from build123d import *

# Parameters (mm, degrees)
F0_W     = 140
F0_H     = 60
F1_DEPTH = 60
F2_R     = 10
F3_DEPTH = 20
F4_R     = 10
F5_DEPTH = 65
F6_R     = 10
F7_DEPTH = 20


with BuildPart() as f1:
    # F0 (on Front) → F1 (new body)
    with BuildSketch(Plane.XZ):
        Rectangle(F0_W, F0_H)
    extrude(amount=F1_DEPTH)

    # F2 (on face) → F3 (join)
    with BuildSketch(Plane.XY.offset(30)):
        with Locations((-40, -30)):
            Circle(F2_R)
    extrude(amount=F3_DEPTH)

    # F4 (on face) → F5 (cut)
    with BuildSketch(Plane.XY.offset(30)):
        with Locations((0, -30)):
            Circle(F4_R)
    extrude(amount=-F5_DEPTH, mode=Mode.SUBTRACT)

    # F6 (on face) → F7 (cut)
    with BuildSketch(Plane.XY.offset(30)):
        with Locations((40, -30)):
            Circle(F6_R)
    extrude(amount=-F7_DEPTH, mode=Mode.SUBTRACT)


solid = f1.part
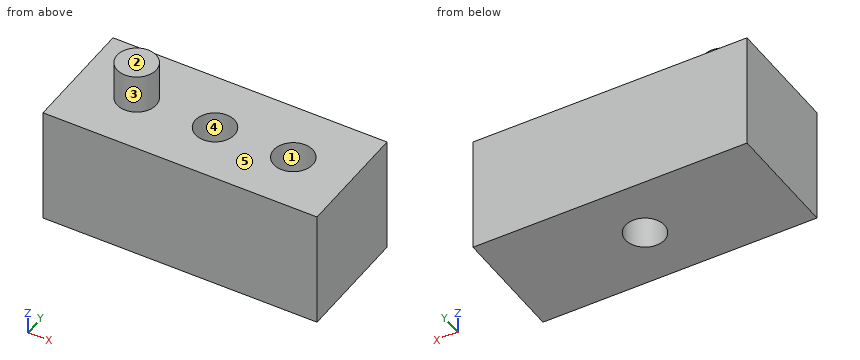
Model file for the job. Use its own axes, mm. Face numbers are marked on the shaded views. A direction names the side the tool comes from. Coordinates: 2 decimals unless noted, no trailing zeros. Write each loop counter-clockwise with the first axis right and the second up, starting at its lowest first coordinate (ties: lowest second). Pieces come first, ordered by that corner, then holes. Notation, with made-up numbers: (19, 79.5) -> (42, 79.5) arc R26 ccw to (42, 102.5) -> close; hole circle Ø10 at (-12, 41.5). An arc over 180 degrees is marked (long way). One line per item, written item: value. Start each with the question number.
1) Probe probe 1 along Y at (x, z) = (40, 19.75); probe 2 along Z at (x, y) = (-47.5, -3); probe 3 along X at (y, z) = (-26, 34). List the from-to ranges inside material, lowest first.
2) Pull direction X, two halves, no side cores. Call the marked faces 3, 4 and 5: +X half, -X half, draft (parallel to the pull), parting line (faces both ways), or undercut.
3) Slice it at B-B on y = -30. Write the cut outline in (x, z), then the cut area to 3 significant figures.
4) Flat gauge pins, fed straight in: pin 1 Ø6 at (x, z) = (28, -14.5) entering from +Y; pin 2 Ø10 at (x, y) = (44.5, -27.5) entering from +Z. Where does each tip first touch, or does it go through?
5) Slice it at D-D on x = -40. Write the cut outline in (y, z).
6) Slice it at C-C on z = 24.5. Write the cut outline in (x, y), then the cut area to 3 significant figures.
7) Which spindle directions (+Z, -Z, +X, -X, +Y, -Y) get a long thin tool onto all of the face, cutting with end or side? Do the marked faces 1 and 2. Say none if no direction does.
8) Slice it at A-A on x = 0. Write the cut outline in (y, z).
Answers follow:
1. probe 1: -60 to -40, -20 to 0
1. probe 2: -30 to 30
1. probe 3: -49.17 to -30.83
2. face 3: parting line
2. face 4: undercut
2. face 5: draft
3. outline: (-70, -30) -> (-10, -30) -> (-10, 30) -> (-30, 30) -> (-30, 50) -> (-50, 50) -> (-50, 30) -> (-70, 30) -> close; (10, -30) -> (70, -30) -> (70, 30) -> (50, 30) -> (50, 10) -> (30, 10) -> (30, 30) -> (10, 30) -> close
3. area: 7,200 mm2
4. pin 1: y = 0
4. pin 2: z = 30
5. outline: (-60, -30) -> (0, -30) -> (0, 30) -> (-20, 30) -> (-20, 50) -> (-40, 50) -> (-40, 30) -> (-60, 30) -> close
6. outline: (-70, -60) -> (70, -60) -> (70, 0) -> (-70, 0) -> close; hole circle Ø20 at (0, -30); hole circle Ø20 at (40, -30)
6. area: 7,770 mm2
7. face 1: +Z
7. face 2: +Z, +X, -X, +Y, -Y
8. outline: (-60, -30) -> (-40, -30) -> (-40, 30) -> (-60, 30) -> close; (-20, -30) -> (0, -30) -> (0, 30) -> (-20, 30) -> close
